Design review of the part built by this model. Coordinates are the model's own, in mm. Round coordinates to 2 decimals unless told otherwise and drop trailing zeros. Loops run counter-clockwise (first coordinate to the right, second up) from the corner with the lowest first, then second, coordinate; pieces in that order, holes last. Notation, with made-up numbers: (59, -13.75) - (97, -13.75) arc R26 cw to (97, 14.25) - close; hole circle Ø10 at (26.5, 77.5). An arc over 180 degrees is marked (long way). One line per question, with ' | ' between items. Start each with the question number.
Autodesk Fusion 360 part; units mm, degrees
sketch "Sketch1" plane through (0, 0, 0) normal (0, 0, 1) x (1, 0, 0)
  line L0 (3.1266, 0.0539) -> (-21.8734, -43.2474)
  line L1 (-21.8734, -43.2474) -> (3.1266, -86.5486)
  line L2 (3.1266, -86.5486) -> (53.1266, -86.5486)
  line L3 (53.1266, -86.5486) -> (78.1266, -43.2474)
  line L4 (78.1266, -43.2474) -> (53.1266, 0.0539)
  line L5 (53.1266, 0.0539) -> (3.1266, 0.0539)
  point P0 (28.1266, -43.2474)
  dimension "d1" = 50
extrude "Extrude1" add sketch "Sketch1" along normal blind 7
sketch "Sketch2" plane through (0, 0, 7) normal (0, 0, 1) x (-1, 0, 0)
  line L0 (-53.1266, -0.0539) -> (-3.1266, -0.0539)
  line L1 (-3.1266, -0.0539) -> (21.8734, 43.2474)
  line L2 (21.8734, 43.2474) -> (-3.1266, 86.5486)
  line L3 (-3.1266, 86.5486) -> (-53.1266, 86.5486)
  line L4 (-53.1266, 86.5486) -> (-78.1266, 43.2474)
  line L5 (-78.1266, 43.2474) -> (-53.1266, -0.0539)
  line L6 (-13.626, 18.1326) -> (-12.126, 20.7307)
  line L7 (-12.126, 20.7307) -> (-13.626, 23.3288)
  line L8 (-13.626, 23.3288) -> (-16.626, 23.3288)
  line L9 (-16.626, 23.3288) -> (-18.126, 20.7307)
  line L10 (-18.126, 20.7307) -> (-16.626, 18.1326)
  line L11 (-16.626, 18.1326) -> (-13.626, 18.1326)
  line L12 (-44.126, 20.7307) -> (-42.626, 18.1326)
  line L13 (-42.626, 18.1326) -> (-39.626, 18.1326)
  line L14 (-39.626, 18.1326) -> (-38.126, 20.7307)
  line L15 (-38.126, 20.7307) -> (-39.626, 23.3288)
  line L16 (-39.626, 23.3288) -> (-42.626, 23.3288)
  line L17 (-42.626, 23.3288) -> (-44.126, 20.7307)
  line L18 (-44.126, 20.7307) -> (-33.8895, 20.7307) construction
  line L19 (-55.626, 40.6493) -> (-52.626, 40.6493)
  line L20 (-52.626, 40.6493) -> (-51.126, 43.2473)
  line L21 (-51.126, 43.2473) -> (-52.626, 45.8454)
  line L22 (-52.626, 45.8454) -> (-55.626, 45.8454)
  line L23 (-55.626, 45.8454) -> (-57.126, 43.2473)
  line L24 (-57.126, 43.2473) -> (-55.626, 40.6493)
  line L25 (-55.626, 40.6493) -> (-56.8973, 40.6493) construction
  line L26 (-38.126, 65.764) -> (-39.626, 68.3621)
  line L27 (-39.626, 68.3621) -> (-42.626, 68.3621)
  line L28 (-42.626, 68.3621) -> (-44.126, 65.764)
  line L29 (-44.126, 65.764) -> (-42.626, 63.1659)
  line L30 (-42.626, 63.1659) -> (-39.626, 63.1659)
  line L31 (-39.626, 63.1659) -> (-38.126, 65.764)
  line L32 (-38.126, 65.764) -> (-41.1962, 65.764) construction
  line L33 (-13.626, 63.1659) -> (-12.126, 65.764)
  line L34 (-12.126, 65.764) -> (-13.626, 68.3621)
  line L35 (-13.626, 68.3621) -> (-16.626, 68.3621)
  line L36 (-16.626, 68.3621) -> (-18.126, 65.764)
  line L37 (-18.126, 65.764) -> (-16.626, 63.1659)
  line L38 (-16.626, 63.1659) -> (-13.626, 63.1659)
  line L39 (-13.626, 63.1659) -> (5.8693, 63.1659) construction
  line L40 (-0.626, 40.6493) -> (0.874, 43.2473)
  line L41 (0.874, 43.2473) -> (-0.626, 45.8454)
  line L42 (-0.626, 45.8454) -> (-3.626, 45.8454)
  line L43 (-3.626, 45.8454) -> (-5.126, 43.2473)
  line L44 (-5.126, 43.2473) -> (-3.626, 40.6493)
  line L45 (-3.626, 40.6493) -> (-0.626, 40.6493)
  line L46 (-0.626, 40.6493) -> (25.3601, 40.6493) construction
  point P0 (-15.126, 20.7307)
  point P1 (-41.126, 20.7307)
  point P2 (-54.126, 43.2473)
  point P3 (-41.126, 65.764)
  point P4 (-15.126, 65.764)
  point P5 (-2.126, 43.2473)
  dimension "d4" = 3
  dimension "d5" = 60
  dimension "d6" = 3
  dimension "d7" = 60
  dimension "d8" = 3
  dimension "d9" = 60
  dimension "d10" = 3
  dimension "d11" = 60
  dimension "d12" = 3
  dimension "d13" = 60
  dimension "d15" = 20
  dimension "d16" = 20
  dimension "d17" = 20
  dimension "d20" = 3
  dimension "d21" = 20
  dimension "d22" = 20
  dimension "d23" = 20
  dimension "d26" = 18.1865
  dimension "d27" = 18.1866
  dimension "d28" = 18.187
  dimension "d29" = 18.187
extrude "Extrude2" cut sketch "Sketch2" against normal blind 5.2 contours L6 L7 L8 L9 L10 L11 | L12 L13 L14 L15 L16 L17 | L19 L20 L21 L22 L23 L24 | L26 L27 L28 L29 L30 L31 | L33 L34 L35 L36 L37 L38 | L40 L41 L42 L43 L44 L45
sketch "Sketch4" plane through (0, 0, 0) normal (0, 0, -1) x (1, 0, 0)
  line L0 (3.1266, -0.0539) -> (53.1266, -0.0539)
  line L1 (53.1266, -0.0539) -> (78.1266, 43.2474)
  line L2 (78.1266, 43.2474) -> (53.1266, 86.5486)
  line L3 (53.1266, 86.5486) -> (3.1266, 86.5486)
  line L4 (3.1266, 86.5486) -> (-21.8734, 43.2474)
  line L5 (-21.8734, 43.2474) -> (3.1266, -0.0539)
  circle A0 centre (28.127, 43.2471) radius 3
  dimension "d38" = 6
  dimension "d39" = 43.3015
  dimension "d40" = 43.3015
  dimension "d41" = 43.3008
extrude "Extrude4" cut sketch "Sketch4" against normal blind 4 contours A0
fillet "Fillet1" radius 1 1 edges at (25.33, -44.332, 0)
1. Clearance check with flat-ended pins moving along their axes: P1, Ø1.6, axis at x = 1, y = -43.5, coming from the +Z side; P2, Ø4, axis at x = -8.5, z = 2.5, coming from the -Y side; P3, Ø3, axis at x = 28.5, y = -44, coming from the -Z side. State where each tip first meets the part, or that it passes through.
2. Take a section at A-A, the plane z = 5.25. Count the separate pieces of the cut face and the enclosed holes in it, then the cut area to 3 significant figures.
3. Take a section at C-C, the plane x = -2.5. Give the boundary of the cut face in (y, z).
4. Take a section at D-D, the plane y = -79. Give the boundary of the cut face in (x, z), then the cut area to 3 significant figures.
5. The part is to be moulded in two halves that separate along Y. For faces 1 (the face through (15, -21, 1.8)), 2 (the face through (28, 0.054, 3)), 3 (the face through (28, -86.549, 3)), say which applies: pulls with the +Y half, pulls with the -Y half, needs draft (parallel to the pull), parting line crosses it, or undercut.
6. Take a section at B-B, the plane y = -22. Give the boundary of the cut face in (x, z).
7. To check wall thickness, follow line 1 along Y through (x, z) = (42.5, 3); line 2 along Y through (x, z) = (3.5, 3); line 3 along X through (y, z) = (-45, 3.5). State the ranges of each line that lie inside material, in increasing order.
Answer list:
1) P1: stops at z = 1.8 | P2: stops at y = -69.87 | P3: stops at z = 4
2) separate pieces: 1 | enclosed holes: 6 | area: 6,350 mm²
3) outline: (-76.8, 0) - (-9.69, 0) - (-9.69, 7) - (-76.8, 7) - close
4) outline: (-1.23, 0) - (57.48, 0) - (57.48, 7) - (-1.23, 7) - close | area: 411 mm²
5) face 1: undercut | face 2: pulls with the +Y half | face 3: pulls with the -Y half
6) outline: (-9.61, 0) - (65.86, 0) - (65.86, 7) - (43.39, 7) - (43.39, 1.8) - (38.86, 1.8) - (38.86, 7) - (17.39, 7) - (17.39, 1.8) - (12.86, 1.8) - (12.86, 7) - (-9.61, 7) - close
7) line 1: y = -86.55 to -68.36, -63.17 to -23.33, -18.13 to 0.05 | line 2: y = -86.55 to -45.85, -40.65 to 0.05 | line 3: x = -20.86 to 0.14, 4.11 to 25.69, 30.56 to 52.14, 56.11 to 77.11
